Here's the drawing with two shaded views (mm, measured from the low corner). I have some questions. A direction names the side the tool comes from. Round coordinates to 2 decimals unless told otherwise and drop trailing zeros. Order: outer loops, then holes, each group sorted by start corner. A loop starts at its lowest first (then second) coordinate and runs counter-clockwise, first axis right, second up.
Q1. If we section it at B-B (y = 3): Please give me the cut outline in (x, z).
Q2. Will these pins go through, and if not, where does the flat tip stop? P1, Ø4.5, axis at y = 11.5, z = 9.5, coming from the -X side; P2, Ø3, axis at x = 32.5, y = 16, coming from the +Z side; P3, Ø2, axis at x = 60, z = 6.5, coming from the +Y side.
Q3. If we section it at C-C (x = 9): Please give me the cut outline in (y, z).
Q4. If I drill on line 1 (Z direction, x = 48, y = 3.5); line 2 (Z direction, x = 57.5, y = 12), over which ranges is the centre line in solid material (lowest first)?
Q5. For the marked faces 1 and 2, which set-ups out of +Z, -Z, +X, -X, +Y, -Y let a thin tool reach every point of the face, with its end or its side?
Q6. If we section it at A-A (z = 4.25): Please give me the cut outline in (x, y), plus the area to 3 significant figures.
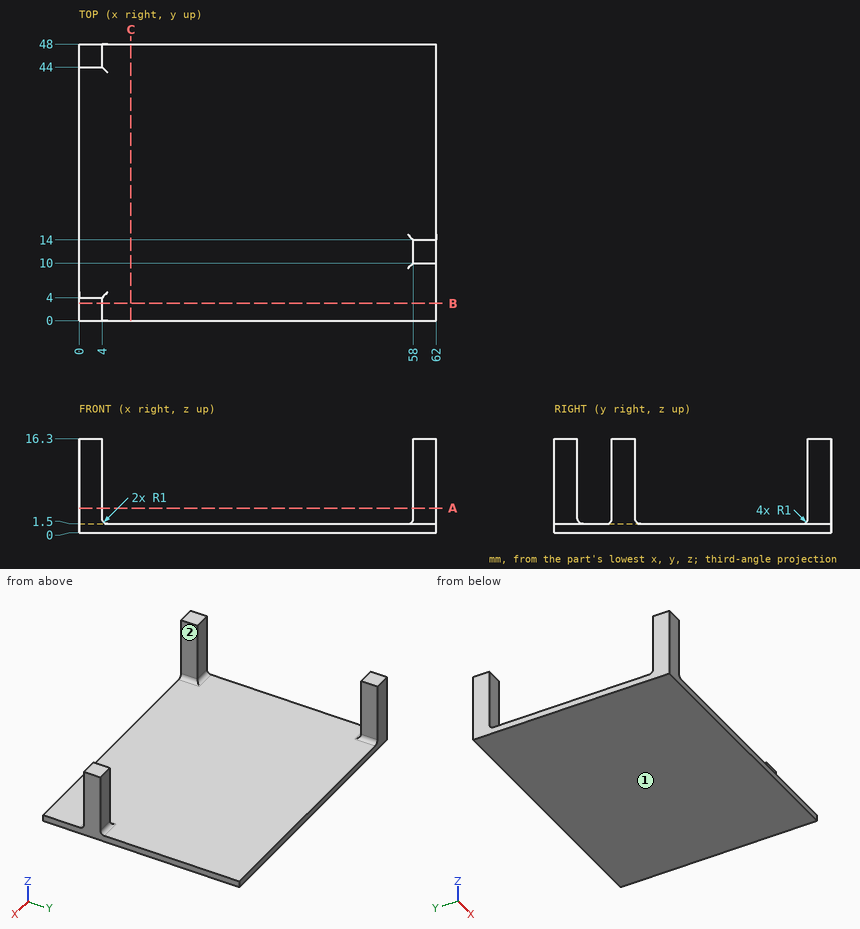
Solution:
1. outline: (0, 0) - (62, 0) - (62, 1.5) - (5, 1.5) arc R1 cw to (4, 2.5) - (4, 16.3) - (0, 16.3) - close
2. P1: stops at x = 58
2. P2: stops at z = 1.5
2. P3: stops at y = 14
3. outline: (0, 0) - (48, 0) - (48, 1.5) - (0, 1.5) - close
4. line 1: z = 0 to 1.5
4. line 2: z = 0 to 1.63
5. face 1: -Z, +X, -X, +Y, -Y
5. face 2: +Z, +X, +Y, -Y
6. outline: (0, 0) - (4, 0) - (4, 4) - (0, 4) - close; (0, 44) - (4, 44) - (4, 48) - (0, 48) - close; (58, 10) - (62, 10) - (62, 14) - (58, 14) - close
6. area: 48.0 mm2
